Autodesk Inventor part; units mm, degrees
ref_plane "YZ Plane" through (0, 0, 0) normal (1, 0, 0) x (0, 1, 0)
ref_plane "XZ Plane" through (0, 0, 0) normal (0, 1, 0) x (-1, 0, 0)
ref_plane "XY Plane" through (0, 0, 0) normal (0, 0, 1) x (1, 0, 0)
sketch "Boceto1" plane through (0, 0, 0) normal (0, 1, 0) x (-1, 0, 0)
  line L0 (0, 0) -> (50, 0)
  line L1 (50, 0) -> (50, -65)
  line L2 (50, -65) -> (0, -65)
  line L3 (0, -65) -> (0, 0)
  line L4 (17.7, -45) -> (32.7, -45)
  line L5 (32.7, -45) -> (32.7, -20)
  line L6 (32.7, -20) -> (17.7, -20)
  line L7 (17.7, -20) -> (17.7, -45)
  line L8 (17.7, -45) -> (32.7, -20) construction
  line L9 (32.7, -45) -> (17.7, -20) construction
  line L10 (35.7, -17) -> (35.7, -48)
  line L11 (35.7, -48) -> (14.7, -48)
  line L12 (14.7, -48) -> (14.7, -17)
  line L13 (14.7, -17) -> (35.7, -17)
  line L14 (41, -1.5) -> (9, -1.5)
  line L15 (9, -1.5) -> (9, -14)
  line L16 (9, -14) -> (41, -14)
  line L17 (41, -14) -> (41, -1.5)
  line L18 (32.7, -32.5) -> (17.7, -32.5) construction
  line L19 (41, -7.75) -> (35.5, -7.75) construction
  line L20 (35.5, -7.75) -> (14.5, -7.75) construction
  line L21 (14.5, -7.75) -> (9, -7.75) construction
  circle A0 centre (35.5, -7.75) radius 1.4
  circle A1 centre (14.5, -7.75) radius 1.4
  line L22 (41, -63.5) -> (9, -63.5)
  line L23 (9, -63.5) -> (9, -51)
  line L24 (9, -51) -> (41, -51)
  line L25 (41, -51) -> (41, -63.5)
  circle A2 centre (35.5, -57.25) radius 1.4
  circle A3 centre (14.5, -57.25) radius 1.4
  line L26 (50, -32.5) -> (43.2, -32.5) construction
  line L27 (0, -32.5) -> (6.8, -32.5)
  line L28 (45.9347, 0) -> (45.9347, -14) construction
  line L29 (43.2, -32.5) -> (43.2, -14.5) construction
  line L30 (43.2, -14.5) -> (50, -14.5) construction
  circle A4 centre (43.2, -14.5) radius 1.4
  line L31 (25.2, -20) -> (25.2, -45) construction
  circle A5 centre (7.2, -14.5) radius 1.4
  circle A6 centre (35.5, -57.25) radius 1.4
  circle A7 centre (43.2, -50.5) radius 1.4
  circle A8 centre (7.2, -50.5) radius 1.4
  line L32 (35.5, -7.75) -> (14.5, -7.75)
  point P0 (25.2, -32.5)
  point P1 (25, -14)
  point P2 (25.2, -17)
  dimension "d0" = 65
  dimension "d1" = 50
  dimension "d2" = 25
  dimension "d3" = 15
  dimension "d4" = 3
  dimension "d5" = 12.5
  dimension "d6" = 32
  dimension "d7" = 3
  dimension "d8" = 5.5
  dimension "d9" = 5.5
  dimension "d10" = 2.8
  dimension "d11" = 2.8
  dimension "d12" = 6.8
  dimension "d13" = 6.8
  dimension "d14" = 14
  dimension "d15" = 2.8
  dimension "d30" = 36
  dimension "d31" = 36
  dimension "d32" = 1.5
extrude "Extrusión1" add sketch "Boceto1" along normal blind 3 contours L10 L11 L12 L13
extrude "Extrusión2" add sketch "Boceto1" against normal blind 4 contours L0 L1 L2 L3 | L17 L16 L15 L14 | L22 L23 L24 L25
extrude "Extrusión3" add sketch "Boceto1" along normal blind 2.5 contours L17 L16 L15 L14 | L22 L23 L24 L25
sketch "Boceto2" plane through (0, 2.5, 0) normal (0, 1, 0) x (1, 0, 0)
  line L0 (-41, 1.5) -> (-9, 1.5)
  line L1 (-25, 1.5) -> (-25, 14)
  line L2 (-9, 14) -> (-41, 14)
  line L3 (-20, 1.5) -> (-30, 1.5)
  line L4 (-30, 1.5) -> (-30, 14)
  line L5 (-30, 14) -> (-20, 14)
  line L6 (-20, 14) -> (-20, 1.5)
  line L7 (-20, 1.5) -> (-30, 14) construction
  line L8 (-30, 1.5) -> (-20, 14) construction
  line L9 (-32.7, 32.5) -> (-17.7, 32.5) construction
  line L10 (-41, 63.5) -> (-9, 63.5)
  line L11 (-9, 51) -> (-41, 51)
  line L12 (-30, 63.5) -> (-30, 51)
  line L13 (-20, 51) -> (-20, 63.5)
  point P0 (0, 0)
  point P1 (-25, 7.75)
  dimension "d22" = 10
extrude "Extrusión4" cut sketch "Boceto2" against normal blind 0.75
extrude "Extrusión5" add sketch "Boceto1" against normal blind 4 contours L7 L6 L5 L4 | L10 L11 L12 L13
sketch "Boceto3" plane through (0, 3, 0) normal (0, 1, 0) x (1, 0, 0)
  line L0 (-25.2, 20) -> (-25.2, 45) construction
  line L1 (-35.7, 17) -> (-14.7, 17)
  line L2 (-25.2, 17) -> (-25.2, 48)
  line L3 (-14.7, 48) -> (-35.7, 48)
  line L4 (-24.95, 17) -> (-25.45, 17)
  line L5 (-25.45, 17) -> (-25.45, 48)
  line L6 (-25.45, 48) -> (-24.95, 48)
  line L7 (-24.95, 48) -> (-24.95, 17)
  line L8 (-24.95, 17) -> (-25.45, 48) construction
  line L9 (-25.45, 17) -> (-24.95, 48) construction
  point P0 (0, 0)
  point P1 (-25.2, 32.5)
  point P2 (-24.95, 17)
  point P3 (-24.95, 48)
  point P4 (-25.45, 17)
  dimension "d27" = 0.5
extrude "Extrusión6" cut sketch "Boceto3" against normal blind 0.5
sketch "Boceto4" plane through (-41, 0, -1.5) normal (0, 0, 1) x (1, 0, 0)
  line L0 (16.05, 2.5) -> (15.55, 2.5)
  line L1 (21, 1.75) -> (11, 1.75)
  line L2 (-9, 0) -> (41, 0)
  line L3 (15.55, 2.5) -> (15.55, 3)
fillet "Empalme1" radius 2 4 edges at (-41, 1.25, -51) (-9, 1.25, -51) (-9, 1.25, -14) (-41, 1.25, -14)
equation "\"d9\" = d8"
equation "\"d13\" = d12"
properties part number "Molde 1FBR 0.5mm"
Can you work these out from the model? Positions are in its coordinate system, mm. A direction names the side the tool comes from. Coordinates: 2 decimals unless noted, no trailing zeros. Loops run counter-clockwise (first coordinate to the right, second up) from the corner with the lowest first, then second, coordinate; pieces in that order, holes last. Notation, with made-up numbers: (10, 29) - (39, 29) arc R11 ccw to (39, 47) - close; hole circle Ø10 at (48.25, 12). An arc over 180 degrees is marked (long way). Put each result on its own line as item: value. Start each with the question number.
Item 1: Suppose I cut it at C-C (y = -3). State how many separate pieces and enclosed holes the cut face has, and give its area (3 significant figures).
Item 2: Suppose I cut it at A-A (x = -43.2). Please give me the cut outline in (y, z), and give its area (3 significant figures).
Item 3: Suppose I cut it at D-D (x = -28). Please give me the cut outline in (y, z), and give its area (3 significant figures).
Item 4: For pin 1 (0.8 mm diameter, centred on y = 2, z = -60, fed in from -X); pin 2 (2 mm diameter, centred on y = 2, z = -57.5, fed in from +X); pin 3 (0.9 mm diameter, centred on x = -24.5, y = 1, fed in from +Z), each with a flat end and sliding along its axis, tell me the tip position at first contact or that it passes through.
Item 5: If I drill on line 1 along Z through (x, y) = (-35.5, -2.25); line 2 along Z through (x, y) = (-43.2, -2.8); line 3 along X through (y, z) = (1, -23.5), over which ranges is the centre line in solid material (lowest first)?
Item 6: Which directions (+Z, -Z, +X, -X, +Y, -Y) give clear straight access to the entire face, cutting with the end or side of a thin tool? Please do faces 1 (the face through (-35.7, 1, -32)), 2 (the face through (-25, 1, -17)), 3 (the face through (-9.57, 1.27, -13.4)).
Item 7: If we mould it in two halves opening along Z, with no side actions, what happens to faces 4 (the face through (-25, 1, -1.5)), 5 (the face through (-25, 1, -51)), 6 (the face through (-16, 2.5, -59))? For each: +Z half, -Z half, draft (parallel to the pull), parting line (faces both ways), or undercut.
Item 8: Suppose I cut it at B-B (z = -7.75). Please give me the cut outline in (x, y).
Here are the results:
1. separate pieces: 1
1. enclosed holes: 8
1. area: 3,200 mm²
2. outline: (-4, -65) - (0, -65) - (0, -51.9) - (-4, -51.9) - close; (-4, -49.1) - (0, -49.1) - (0, -15.9) - (-4, -15.9) - close; (-4, -13.1) - (0, -13.1) - (0, 0) - (-4, 0) - close
2. area: 238 mm²
3. outline: (-4, -65) - (0, -65) - (0, -63.5) - (1.75, -63.5) - (1.75, -51) - (0, -51) - (0, -48) - (3, -48) - (3, -45) - (0, -45) - (0, -20) - (3, -20) - (3, -17) - (0, -17) - (0, -14) - (1.75, -14) - (1.75, -1.5) - (0, -1.5) - (0, 0) - (-4, 0) - close
3. area: 322 mm²
4. pin 1: x = -41
4. pin 2: x = -9
4. pin 3: z = -1.5
5. line 1: -65 to -58.65, -55.85 to -9.15, -6.35 to 0
5. line 2: -65 to -51.9, -49.1 to -15.9, -13.1 to 0
5. line 3: -35.7 to -32.7, -17.7 to -14.7
6. face 1: -X, +Y
6. face 2: +X, -X, +Y
6. face 3: +X, +Y
7. face 4: +Z half
7. face 5: undercut
7. face 6: draft
8. outline: (-50, -4) - (-36.9, -4) - (-36.9, 2.5) - (-41, 2.5) - (-41, 0) - (-50, 0) - close; (-34.1, -4) - (-15.9, -4) - (-15.9, 2.5) - (-20, 2.5) - (-20, 1.75) - (-30, 1.75) - (-30, 2.5) - (-34.1, 2.5) - close; (-13.1, -4) - (0, -4) - (0, 0) - (-9, 0) - (-9, 2.5) - (-13.1, 2.5) - close
